The listing builds one solid part. Answer for the finished solid, in the listing's coordinates (mm). Give positions to 0.01 mm unless a question says otherwise; leave off trailing zeros. Write each loop counter-clockwise with the first axis right and the second up, starting at its lowest first coordinate (ties: lowest second). Pieces come first, ordered by that corner, then holes. Notation, with made-up numbers: (79, -25.75) - (121, -25.75) arc R24 ccw to (121, 3.25) - close; hole circle Ø10 at (31, -31.75). An arc over 180 degrees is marked (long way). Answer as CSV lines item,"result". Start each with the question number.
(1) Find section D-D (x = -31.75). Write down the section's boundary in (y, z).
(2) Find section A-A (x = 0). State how many separate pieces and enclosed holes the cut face has, then the cut area to 3 significant figures.
(3) Find section C-C (x = -76.5). Write down the section's boundary in (y, z).
(4) Straight lines are drawn through the part: probe 1 along Z at (x, y) = (-51, 3.75); probe 2 along Z at (x, y) = (20.5, 3). For each, find the intervals that lie inside material, in ascending order.
(5) For a pull along Z with two mould halves and no side action, classify faces 1 (the face through (0.553, 4.186, 29.258)), 2 (the face through (84.795, 3.131, -26.703)), 3 (the face through (-1, 0, 19)) as pulls with the +Z half, pulls with the -Z half, needs draft (parallel to the pull), parting line crosses it, or undercut.
from build123d import *

# Parameters (mm, degrees)
SKETCH1_R                                          = 88.9
SKETCH1_R_2                                        = 6.35
BOSS_EXTRUDE1_DEPTH                                = 6.35
CSK_FOR_10_FLAT_HEAD_MACHINE_SCREW_100_D           = 5.1054
CSK_FOR_10_FLAT_HEAD_MACHINE_SCREW_100_CSINK_D     = 9.779
CSK_FOR_10_FLAT_HEAD_MACHINE_SCREW_100_CSINK_ANGLE = 100
F_1_4_0_25_DIAMETER_HOLE1_D                        = 6.35
CIRPATTERN1_COUNT                                  = 8


with BuildPart() as part:
    # Sketch1 → Boss-Extrude1 (new body)
    with BuildSketch(Plane(origin=(0, 0, 0), x_dir=(1, 0, 0), z_dir=(0, 1, 0))):
        Circle(SKETCH1_R)
        Circle(SKETCH1_R_2, mode=Mode.SUBTRACT)
    extrude(amount=BOSS_EXTRUDE1_DEPTH)

    # CSK for #10 Flat Head Machine Screw (100)1 (through all)
    with Locations(Plane(origin=(31.75, 0, 0), x_dir=(0, 0, -1), z_dir=(0, -1, 0))):
        with Locations((0, 0)):
            csk_for_10_flat_head_machine_screw_100 = CounterSinkHole(CSK_FOR_10_FLAT_HEAD_MACHINE_SCREW_100_D / 2, CSK_FOR_10_FLAT_HEAD_MACHINE_SCREW_100_CSINK_D / 2, counter_sink_angle=CSK_FOR_10_FLAT_HEAD_MACHINE_SCREW_100_CSINK_ANGLE)

    # 1/4 (0.25) Diameter Hole1 (through all)
    with Locations(Plane(origin=(0, 6.35, 0), x_dir=(1, 0, 0), z_dir=(0, 1, 0))):
        with Locations((76.2, 0)):
            f_1_4_0_25_diameter_hole1 = Hole(F_1_4_0_25_DIAMETER_HOLE1_D / 2)

    # CirPattern1: CSK for #10 Flat Head Machine Screw (100)1, 1/4 (0.25) Diameter Hole1 ×8 about axis
    cirpattern1_axis = Axis((0, 0, 0), (0, 1, 0))
    for i in range(1, CIRPATTERN1_COUNT):
        add(csk_for_10_flat_head_machine_screw_100.rotate(cirpattern1_axis, i * 360 / CIRPATTERN1_COUNT), mode=Mode.SUBTRACT)
        add(f_1_4_0_25_diameter_hole1.rotate(cirpattern1_axis, i * 360 / CIRPATTERN1_COUNT), mode=Mode.SUBTRACT)


solid = part.part
Result set:
1,outline,"(0, -83.04) - (6.35, -83.04) - (6.35, -2.55) - (1.96, -2.55) - (0, -4.89) - close; (0, 4.89) - (1.96, 2.55) - (6.35, 2.55) - (6.35, 83.04) - (0, 83.04) - close"
2,separate pieces,"6"
2,enclosed holes,"0"
2,area,"894 mm^2"
3,outline,"(0, -45.29) - (6.35, -45.29) - (6.35, -3.16) - (0, -3.16) - close; (0, 3.16) - (6.35, 3.16) - (6.35, 45.29) - (0, 45.29) - close"
4,probe 1,"-72.82 to -55.21, -52.55 to 52.55, 55.21 to 72.82"
4,probe 2,"-86.5 to -24.1, -20.8 to 20.8, 24.1 to 86.5"
5,face 1,"undercut"
5,face 2,"parting line crosses it"
5,face 3,"needs draft"
